Input: dimensioned drawing with shaded views. Units: mm. Origin: part minimum x, y, z. Round coordinates to 2 decimals unless told otherwise and drop trailing zeros. Loops run counter-clockwise (first coordinate to the right, second up) from the corner with the lowest first, then second, coordinate; pieces in that order, holes last. Notation, with made-up numbers: (11.5, 79.25) -> (19.5, 79.25) arc R26 ccw to (19.5, 98.25) -> close; hole circle Ø3 at (7, 84). An arc over 180 degrees is marked (long way). Answer as a JSON object with one key per item and string values.
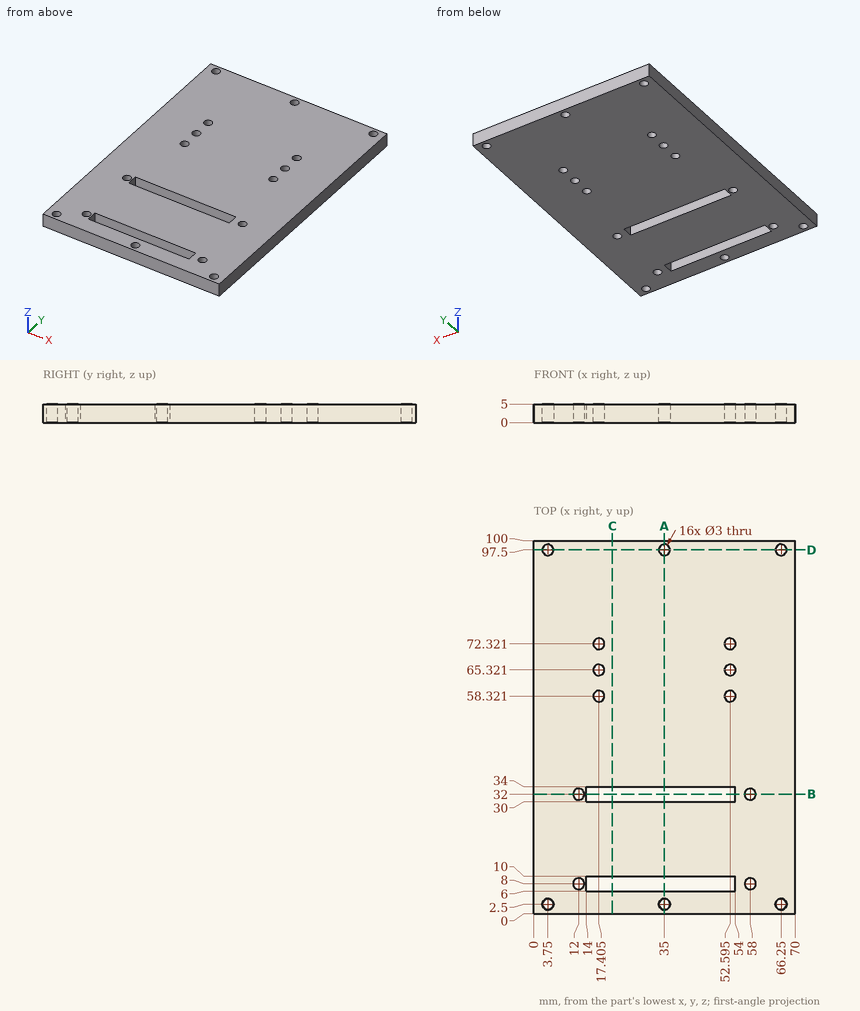
1) Section C-C, the plane x = 21. Output: boundary loops of the cut face in (y, z), plus the area to 3 significant figures.
Output:
{"outline": "(0, 0) -> (6, 0) -> (6, 5) -> (0, 5) -> close; (10, 0) -> (30, 0) -> (30, 5) -> (10, 5) -> close; (34, 0) -> (100, 0) -> (100, 5) -> (34, 5) -> close", "area": "460 mm^2"}
2) Section A-A, the plane x = 35. Output: boundary loops of the cut face in (y, z), plus the area to 3 significant figures.
Output:
{"outline": "(0, 0) -> (1, 0) -> (1, 5) -> (0, 5) -> close; (4, 0) -> (6, 0) -> (6, 5) -> (4, 5) -> close; (10, 0) -> (30, 0) -> (30, 5) -> (10, 5) -> close; (34, 0) -> (96, 0) -> (96, 5) -> (34, 5) -> close; (99, 0) -> (100, 0) -> (100, 5) -> (99, 5) -> close", "area": "430 mm^2"}
3) Section D-D, the plane y = 97.5. Output: boundary loops of the cut face in (x, z).
Output:
{"outline": "(0, 0) -> (2.25, 0) -> (2.25, 5) -> (0, 5) -> close; (5.25, 0) -> (33.5, 0) -> (33.5, 5) -> (5.25, 5) -> close; (36.5, 0) -> (64.75, 0) -> (64.75, 5) -> (36.5, 5) -> close; (67.75, 0) -> (70, 0) -> (70, 5) -> (67.75, 5) -> close"}
4) Contact query for a flat-ended pin moving along its axis: P1, Ø2.5, axis at x = 17.41, y = 58.32, coming from the +Z side. Output: stop coordinate, or through.
Output:
{"P1": "passes through"}
5) Ray query, probe 1 along Y at (x, z) = (66.25, 3.75); probe 2 along Y at (x, z) = (30.5, 2.55); probe 3 along X at (y, z) = (2.5, 1.5). Return the intervals inside material, ascending.
Output:
{"probe 1": "y = 0 to 1, 4 to 96, 99 to 100", "probe 2": "y = 0 to 6, 10 to 30, 34 to 100", "probe 3": "x = 0 to 2.25, 5.25 to 33.5, 36.5 to 64.75, 67.75 to 70"}
6) Section B-B, the plane y = 32. Output: boundary loops of the cut face in (x, z).
Output:
{"outline": "(0, 0) -> (10.5, 0) -> (10.5, 5) -> (0, 5) -> close; (13.5, 0) -> (14, 0) -> (14, 5) -> (13.5, 5) -> close; (54, 0) -> (56.5, 0) -> (56.5, 5) -> (54, 5) -> close; (59.5, 0) -> (70, 0) -> (70, 5) -> (59.5, 5) -> close"}
